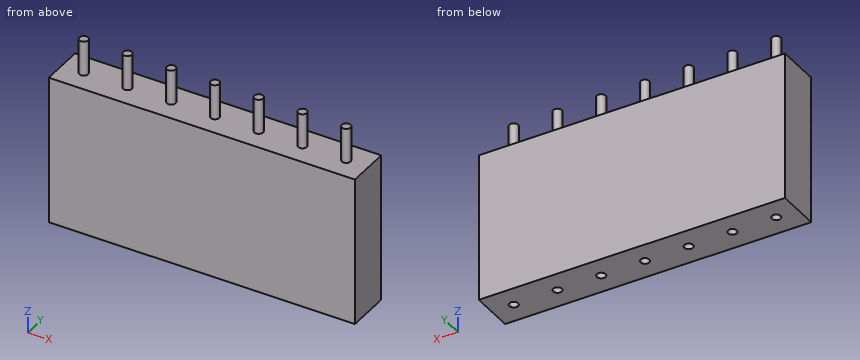
```python
from build123d import *

# Parameters (mm, degrees)
ESQUISSE1_W                = 2.5
ESQUISSE1_H                = 2.5
BOSS_EXTRU_1_DEPTH         = 8.5
ESQUISSE2_R                = 0.25
BOSS_EXTRU_2_DEPTH         = 2
ESQUISSE3_R                = 0.25
ENL_V_MAT_EXTRU_2_DEPTH    = 4
R_P_TITION_LIN_AIRE1_COUNT = 7
R_P_TITION_LIN_AIRE1_PITCH = 2.5


with BuildPart() as part:
    # Esquisse1 → Boss.-Extru.1 (new body)
    with BuildSketch(Plane.XY):
        with Locations((-1.25, 1.25)):
            Rectangle(ESQUISSE1_W, ESQUISSE1_H)
    boss_extru_1 = extrude(amount=BOSS_EXTRU_1_DEPTH)

    # Esquisse2 → Boss.-Extru.2 (add)
    with BuildSketch(Plane.XY.offset(8.5)):
        with Locations((-1.25, 1.25)):
            Circle(ESQUISSE2_R)
    boss_extru_2 = extrude(amount=BOSS_EXTRU_2_DEPTH)

    # Esquisse3 → Enlèv. mat.-Extru.2 (cut)
    with BuildSketch(Plane(origin=(0, 0, 0), x_dir=(-1, 0, 0), z_dir=(0, 0, -1))):
        with Locations(Location((1.25, 1.25, 0), (0, 0, 180))):
            Circle(ESQUISSE3_R)
    enl_v_mat_extru_2 = extrude(amount=-ENL_V_MAT_EXTRU_2_DEPTH, mode=Mode.SUBTRACT)

    # Répétition linéaire1: Boss.-Extru.1, Boss.-Extru.2, Enlèv. mat.-Extru.2 ×7
    with Locations(*[(-i * R_P_TITION_LIN_AIRE1_PITCH, 0, 0) for i in range(1, R_P_TITION_LIN_AIRE1_COUNT)]):
        add(boss_extru_1)
        add(boss_extru_2)
        add(enl_v_mat_extru_2, mode=Mode.SUBTRACT)


solid = part.part
```
Read the model definition and answer for the solid it produces. Units are mm, in the model's axes. Give positions to 0.01 mm unless a question says otherwise; leave off trailing zeros. Write each loop counter-clockwise with the first axis right and the second up, starting at its lowest first coordinate (ties: lowest second). Pieces come first, ordered by that corner, then holes. Notation, with made-up numbers: M 26,65 L 75,65 A24 cw 75,100 Z; hole C -39.75,-19.5 d10. An arc over 180 degrees is marked long. Put each result on its own line as item: value. Start each with the question number.
1. Consider line 1 along Y through (x, z) = (-3.75, 2.75); line 2 along Z through (x, y) = (-7, 1.75). Determine where each line is inside the solid, lowest interval first.
2. The part is cut by section A-A, the plane z = 9.75. Give the vertices of the cut face in (x, y).
3. The part is cut by section C-C, the plane x = -11.25. Give the vertices of the cut face in (y, z), and give its area (4 significant figures).
4. The part is cut by section B-B, the plane z = 1.25. Give the vertices of the cut face in (x, y).
5. This flat-tipped pin is pushed along its axis until it touches: pin 1 Ø0.6 at (x, y) = (-6, 1) entering from -Z. Where does it stop, or does it pass through?
6. The part is cut by section D-D, the plane y = 0.75. Give the vertices of the cut face in (x, z), and give its area (3 significant figures).
Final values:
1. line 1: y = 0 to 1, 1.5 to 2.5
1. line 2: z = 0 to 8.5
2. outline: C -16.25,1.25 d0.5; C -13.75,1.25 d0.5; C -11.25,1.25 d0.5; C -8.75,1.25 d0.5; C -6.25,1.25 d0.5; C -3.75,1.25 d0.5; C -1.25,1.25 d0.5
3. outline: M 0,0 L 1,0 L 1,4 L 1.5,4 L 1.5,0 L 2.5,0 L 2.5,8.5 L 1.5,8.5 L 1.5,10.5 L 1,10.5 L 1,8.5 L 0,8.5 Z
3. area: 20.25 mm²
4. outline: M -17.5,0 L 0,0 L 0,2.5 L -17.5,2.5 Z; hole C -16.25,1.25 d0.5; hole C -13.75,1.25 d0.5; hole C -11.25,1.25 d0.5; hole C -8.75,1.25 d0.5; hole C -6.25,1.25 d0.5; hole C -3.75,1.25 d0.5; hole C -1.25,1.25 d0.5
5. pin 1: stops at z = 0
6. outline: M -17.5,0 L 0,0 L 0,8.5 L -17.5,8.5 Z
6. area: 149 mm²
